Part model, mm, in its own coordinate system. Coordinates: 2 decimals unless noted, no trailing zeros. Loops run counter-clockwise (first coordinate to the right, second up) from the corner with the lowest first, then second, coordinate; pieces in that order, holes last. Notation, with made-up numbers: (46, -25) -> (67, -25) arc R32 cw to (67, 6) -> close; hole circle Ø8 at (-23.75, -21.75). An arc over 180 degrees is marked (long way). One line per question, with ' | ' between items. Start each with the question number.
1) Cut at C-C (x = -13). List the corners of the cut face in (y, z), plus the area to 3 significant figures.
2) Cut at B-B (y = 0). List the corners of the cut face in (x, z), plus the area to 3 significant figures.
3) Cut at D-D (y = -17.5). List the corners of the cut face in (x, z), plus the area to 3 significant figures.
4) Drop flat-ended pins along their axis: pin 1 (1 mm diameter, centred on y = 22, z = 1, fed in from -X); pin 2 (1.5 mm diameter, centred on y = -23, z = 2.5, fed in from +X). Give the stop position or say it passes through.
5) Cut at A-A (x = 0). List the corners of the cut face in (y, z), plus the area to 3 significant figures.
6) Two-plate mould, pull along X, no slides. Class faces 1 (the face through (-32.52, 15.47, 1.48)), 2 (the face through (-9, -40, 1)), 3 (the face through (18, 1, 0)): released by +X, released by -X, zero draft, split by the parting line, or undercut.
7) Probe L1, parallel to Y at x = 0, z = 0.9; L2, parallel to X at y = 18, z = 2.35; L3, parallel to X at y = -36, z = 0.65. List the from-to ranges inside material, lowest first. Write a range as from..to.
from build123d import *

# Parameters (mm, degrees)
SKETCH1_R           = 41
BOSS_EXTRUDE1_DEPTH = 3
SKETCH3_R           = 3
CUT_EXTRUDE1_DEPTH  = 4
CIRPATTERN1_COUNT   = 6
CUT_EXTRUDE2_REACH  = 5
SKETCH4_R           = 16


with BuildPart() as part:
    # Sketch1 → Boss-Extrude1 (new body)
    with BuildSketch(Plane.XY):
        Circle(SKETCH1_R)
    extrude(amount=BOSS_EXTRUDE1_DEPTH)

    # Sketch3 → Cut-Extrude1 (cut, through all)
    with BuildSketch(Plane(origin=(0, 0, 0), x_dir=(-1, 0, 0), z_dir=(0, 0, -1))):
        with Locations((0, 35)):
            Circle(SKETCH3_R)
    cut_extrude1 = extrude(amount=-CUT_EXTRUDE1_DEPTH, mode=Mode.SUBTRACT)

    # CirPattern1: Cut-Extrude1 ×6 about axis
    cirpattern1_axis = Axis((0, 0, 0), (0, 0, 1))
    for i in range(1, CIRPATTERN1_COUNT):
        add(cut_extrude1.rotate(cirpattern1_axis, i * 360 / CIRPATTERN1_COUNT), mode=Mode.SUBTRACT)

    # Sketch4 → Cut-Extrude2 (cut, up to next)
    with BuildSketch(Plane.XY.offset(3), mode=Mode.PRIVATE) as cut_extrude2_sk1:
        Circle(SKETCH4_R)
    cut_extrude2_tool1 = extrude(cut_extrude2_sk1.sketch, amount=-CUT_EXTRUDE2_REACH, mode=Mode.PRIVATE) & part.part
    add(cut_extrude2_tool1.solids().sort_by_distance((0, 0, 3))[0], mode=Mode.SUBTRACT)


solid = part.part
Reported:
1) outline: (-38.88, 0) -> (-9.33, 0) -> (-9.33, 3) -> (-38.88, 3) -> close; (9.33, 0) -> (38.88, 0) -> (38.88, 3) -> (9.33, 3) -> close | area: 177 mm²
2) outline: (-41, 0) -> (-16, 0) -> (-16, 3) -> (-41, 3) -> close; (16, 0) -> (41, 0) -> (41, 3) -> (16, 3) -> close | area: 150 mm²
3) outline: (-37.08, 0) -> (-33.31, 0) -> (-33.31, 3) -> (-37.08, 3) -> close; (-27.31, 0) -> (27.31, 0) -> (27.31, 3) -> (-27.31, 3) -> close; (33.31, 0) -> (37.08, 0) -> (37.08, 3) -> (33.31, 3) -> close | area: 186 mm²
4) pin 1: stops at x = -34.91 | pin 2: stops at x = 34.44
5) outline: (-41, 0) -> (-38, 0) -> (-38, 3) -> (-41, 3) -> close; (-32, 0) -> (-16, 0) -> (-16, 3) -> (-32, 3) -> close; (16, 0) -> (32, 0) -> (32, 3) -> (16, 3) -> close; (38, 0) -> (41, 0) -> (41, 3) -> (38, 3) -> close | area: 114 mm²
6) face 1: undercut | face 2: split by the parting line | face 3: zero draft
7) L1: y = -41..-38, -32..-16, 16..32, 38..41 | L2: x = -36.84..-33.27, -27.35..27.35, 33.27..36.84 | L3: x = -19.62..-2.83, 2.83..19.62
